Source: CAD feature listing. Evaluate the final solid. Frame: model axes, mm. Face numbers are marked on the shaded views. A direction names the side the tool comes from. Give positions to 0.01 mm unless a question says otherwise; leave off trailing zeros. Loops run counter-clockwise (first coordinate to the right, second up) from the corner with the lowest first, then second, coordinate; pieces in that order, holes last. Notation, with made-up numbers: (-21, 21) -> (7, 21) arc R15 ccw to (7, 28) -> close; hole circle Ø9 at (53.5, -35.75). An arc over 180 degrees is marked (long way). Put each result on its own line as item: value.
```python
from build123d import *

# Parameters (mm, degrees)
SKETCH1_R           = 4.05
BOSS_EXTRUDE1_DEPTH = 6.7
SKETCH2_R           = 5.75
SKETCH2_R_2         = 4.05
BOSS_EXTRUDE2_DEPTH = 1.7


with BuildPart() as part:
    # Sketch1 → Boss-Extrude1 (new body)
    with BuildSketch(Plane(origin=(0, 0, 0), x_dir=(1, 0, 0), z_dir=(0, 1, 0))):
        Polygon((3.167381974, -0.528493855), (3.167381974, 6.572914456), (-2.982618026, 10.123618611), (-9.132618026, 6.572914456), (-9.132618026, -0.528493855), (-2.982618026, -4.079198011), align=None)
        with Locations((-2.982618026, 3.0222103)):
            Circle(SKETCH1_R, mode=Mode.SUBTRACT)
    extrude(amount=BOSS_EXTRUDE1_DEPTH)

    # Sketch2 → Boss-Extrude2 (add)
    with BuildSketch(Plane(origin=(0, 6.7, 0), x_dir=(1, 0, 0), z_dir=(0, 1, 0))):
        with Locations((-2.982618026, 3.0222103)):
            Circle(SKETCH2_R)
        with Locations((-2.982618026, 3.0222103)):
            Circle(SKETCH2_R_2, mode=Mode.SUBTRACT)
    extrude(amount=BOSS_EXTRUDE2_DEPTH)


solid = part.part
```
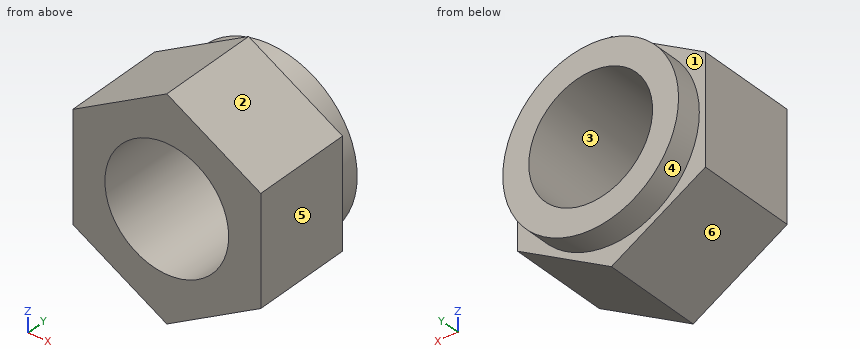
(1) Section D-D on x = -7.5. Return loops of the section in (y, z).
Calculated:
outline: (0, -7.52) -> (6.7, -7.52) -> (6.7, -6.58) -> (8.4, -6.58) -> (8.4, 0.54) -> (6.7, 0.54) -> (6.7, 1.47) -> (0, 1.47) -> close
(2) Draft query along Z for the marked faces 3, 4, 5 and 6. Return one class per face: released by +Z, released by -Z, zero draft, split by the parting line, or undercut.
Calculated:
face 3: undercut
face 4: split by the parting line
face 5: zero draft
face 6: released by -Z
(3) Section C-C on y = 6. Return loops of the section in (x, z), then the cut area to 3 significant figures.
Calculated:
outline: (-9.13, -6.57) -> (-2.98, -10.12) -> (3.17, -6.57) -> (3.17, 0.53) -> (-2.98, 4.08) -> (-9.13, 0.53) -> close; hole circle Ø8.1 at (-2.98, -3.02)
area: 79.5 mm²
(4) Line query: probe 1 along Y at (x, z) = (1.25, -7.25); probe 2 along Z at (x, y) = (0.75, 3.25); probe 3 along Z at (x, y) = (-1.25, 7). Output: solid intervals per line, ascending. Write a range as from..to.
Calculated:
probe 1: y = 0..6.7
probe 2: z = -7.97..-4.59, -1.45..1.92
probe 3: z = -8.5..-6.68, 0.64..2.46
(5) Reachability of the marked faces 1 and 2 from +Z, -Z, +X, -X, +Y, -Y: full face, straight path, thin tool, end or side. Return the list, or none.
Calculated:
face 1: +Y
face 2: +Z, +X, +Y, -Y
(6) First-contact query: P1, Ø1.5, axis at x = -1, z = -3, coming from the +Y side. Flat tip, straight axial feed; report the tip coordinate or a pass-through.
Calculated:
P1: passes through
(7) Section A-A on z = -1.25. Return loops of the section in (x, y).
Calculated:
outline: (-9.13, 0) -> (-6.62, 0) -> (-6.62, 8.4) -> (-8.45, 8.4) -> (-8.45, 6.7) -> (-9.13, 6.7) -> close; (0.66, 0) -> (3.17, 0) -> (3.17, 6.7) -> (2.49, 6.7) -> (2.49, 8.4) -> (0.66, 8.4) -> close
(8) Section B-B on x = -5.25. Return loops of the section in (y, z).
Calculated:
outline: (0, -8.81) -> (6.7, -8.81) -> (6.7, -8.31) -> (8.4, -8.31) -> (8.4, -6.38) -> (0, -6.38) -> close; (0, 0.33) -> (8.4, 0.33) -> (8.4, 2.26) -> (6.7, 2.26) -> (6.7, 2.77) -> (0, 2.77) -> close
